The model under review builds one solid part; all positions refer to its coordinate system, in mm. A direction names the side the tool comes from. Coordinates: 2 decimals unless noted, no trailing zeros. Loops run counter-clockwise (first coordinate to the right, second up) from the corner with the lowest first, then second, coordinate; pieces in that order, holes last. Notation, with made-up numbers: M 85.5,-4.75 L 127.5,-4.75 A18 cw 127.5,9.25 Z; hole C 80,12 d6. An arc over 180 degrees is marked long. One line per item, written item: value.
```python
from build123d import *

# Parameters (mm, degrees)
SKETCH_1_W          = 32
SKETCH_1_H          = 35
EXTRUDE_1_DEPTH     = 14
CUT_EXTRUDE_1_REACH = 37
SKETCH_2_R          = 6.1
EXTRUDE_2_DEPTH     = 33
FILLET_1_R          = 3
SKETCH_6_W          = 14
SKETCH_6_H          = 35
EXTRUDE_4_DEPTH     = 4
CUT_EXTRUDE_2_DEPTH = 10
SKETCH_5_W          = 32
SKETCH_5_H          = 4
EXTRUDE_5_DEPTH     = 2
CUT_EXTRUDE_3_REACH = 20
SKETCH_8_R          = 2
CUT_EXTRUDE_4_DEPTH = 3.5


with BuildPart() as part:
    # Эскиз1 → Бобышка-Вытянуть1 (new body)
    with BuildSketch(Plane.XY):
        Rectangle(SKETCH_1_W, SKETCH_1_H)
    extrude(amount=EXTRUDE_1_DEPTH)

    # Эскиз2 → Вырез-Вытянуть1 (cut, up to next)
    with BuildSketch(Plane(origin=(0, 17.5, 0), x_dir=(1, 0, 0), z_dir=(0, 1, 0)), mode=Mode.PRIVATE) as cut_extrude_1_sk1:
        with Locations((-9, -7)):
            Circle(SKETCH_2_R)
    cut_extrude_1_tool1 = extrude(cut_extrude_1_sk1.sketch, amount=-CUT_EXTRUDE_1_REACH, mode=Mode.PRIVATE) & part.part
    add(cut_extrude_1_tool1.solids().sort_by_distance((-9, 17.5, 7))[0], mode=Mode.SUBTRACT)
    # Эскиз2 → Вырез-Вытянуть1 (cut, up to next)
    with BuildSketch(Plane(origin=(0, 17.5, 0), x_dir=(1, 0, 0), z_dir=(0, 1, 0)), mode=Mode.PRIVATE) as cut_extrude_1_sk2:
        with Locations((9, -7)):
            Circle(SKETCH_2_R)
    cut_extrude_1_tool2 = extrude(cut_extrude_1_sk2.sketch, amount=-CUT_EXTRUDE_1_REACH, mode=Mode.PRIVATE) & part.part
    add(cut_extrude_1_tool2.solids().sort_by_distance((9, 17.5, 7))[0], mode=Mode.SUBTRACT)

    # Эскиз3 → Бобышка-Вытянуть2 (add)
    with BuildSketch(Plane(origin=(0, -17.5, 0), x_dir=(1, 0, 0), z_dir=(0, 1, 0))):
        Polygon((-14, -18), (-10, -14), (10, -14), (14, -18), align=None)
    extrude(amount=EXTRUDE_2_DEPTH)

    # Скругление1
    fillet_1_edges = [part.edges().sort_by_distance(p)[0] for p in [
        (-16, 0, 0),
    ]]
    fillet(fillet_1_edges, radius=FILLET_1_R)

    # Эскиз6 → Бобышка-Вытянуть4 (add)
    with BuildSketch(Plane(origin=(16, 0, 0), x_dir=(0, 0, -1), z_dir=(1, 0, 0))):
        with Locations((-7, 0)):
            Rectangle(SKETCH_6_W, SKETCH_6_H)
    extrude(amount=EXTRUDE_4_DEPTH)

    # Эскиз7 → Вырез-Вытянуть2 (cut)
    with BuildSketch(Plane.XY.offset(14)):
        with BuildLine():
            Line((16, -17.5), (17.5, -17.5))
            ThreePointArc((17.5, -17.5), (18, -17), (17.5, -16.5))
            ThreePointArc((17.5, -16.5), (17, -16), (17.5, -15.5))
            ThreePointArc((17.5, -15.5), (18, -15), (17.5, -14.5))
            ThreePointArc((17.5, -14.5), (17, -14), (17.5, -13.5))
            ThreePointArc((17.5, -13.5), (18, -13), (17.5, -12.5))
            ThreePointArc((17.5, -12.5), (17, -12), (17.5, -11.5))
            ThreePointArc((17.5, -11.5), (18, -11), (17.5, -10.5))
            ThreePointArc((17.5, -10.5), (17, -10), (17.5, -9.5))
            ThreePointArc((17.5, -9.5), (18, -9), (17.5, -8.5))
            ThreePointArc((17.5, -8.5), (17, -8), (17.5, -7.5))
            ThreePointArc((17.5, -7.5), (18, -7), (17.5, -6.5))
            ThreePointArc((17.5, -6.5), (17, -6), (17.5, -5.5))
            ThreePointArc((17.5, -5.5), (18, -5), (17.5, -4.5))
            ThreePointArc((17.5, -4.5), (17, -4), (17.5, -3.5))
            ThreePointArc((17.5, -3.5), (18, -3), (17.5, -2.5))
            ThreePointArc((17.5, -2.5), (17, -2), (17.5, -1.5))
            ThreePointArc((17.5, -1.5), (18, -1), (17.5, -0.5))
            ThreePointArc((17.5, -0.5), (17, 0), (17.5, 0.5))
            ThreePointArc((17.5, 0.5), (18, 1), (17.5, 1.5))
            ThreePointArc((17.5, 1.5), (17, 2), (17.5, 2.5))
            ThreePointArc((17.5, 2.5), (18, 3), (17.5, 3.5))
            ThreePointArc((17.5, 3.5), (17, 4), (17.5, 4.5))
            ThreePointArc((17.5, 4.5), (18, 5), (17.5, 5.5))
            ThreePointArc((17.5, 5.5), (17, 6), (17.5, 6.5))
            ThreePointArc((17.5, 6.5), (18, 7), (17.5, 7.5))
            ThreePointArc((17.5, 7.5), (17, 8), (17.5, 8.5))
            ThreePointArc((17.5, 8.5), (18, 9), (17.5, 9.5))
            ThreePointArc((17.5, 9.5), (17, 10), (17.5, 10.5))
            ThreePointArc((17.5, 10.5), (18, 11), (17.5, 11.5))
            ThreePointArc((17.5, 11.5), (17, 12), (17.5, 12.5))
            ThreePointArc((17.5, 12.5), (18, 13), (17.5, 13.5))
            ThreePointArc((17.5, 13.5), (17, 14), (17.5, 14.5))
            ThreePointArc((17.5, 14.5), (18, 15), (17.5, 15.5))
            ThreePointArc((17.5, 15.5), (17, 16), (17.5, 16.5))
            ThreePointArc((17.5, 16.5), (18, 17), (17.5, 17.5))
            Line((17.5, 17.5), (16, 17.5))
            Line((16, 17.5), (16, -17.5))
        make_face()
    extrude(amount=-CUT_EXTRUDE_2_DEPTH, mode=Mode.SUBTRACT)

    # Эскиз5 → Бобышка-Вытянуть5 (add)
    with BuildSketch(Plane(origin=(0, 15.5, 0), x_dir=(-1, 0, 0), z_dir=(0, 1, 0))):
        with Locations((0, 16)):
            Rectangle(SKETCH_5_W, SKETCH_5_H)
    extrude(amount=EXTRUDE_5_DEPTH)

    # Эскиз8 → Вырез-Вытянуть3 (cut, up to next)
    with BuildSketch(Plane.XY.offset(18), mode=Mode.PRIVATE) as cut_extrude_3_sk1:
        Circle(SKETCH_8_R)
    cut_extrude_3_tool1 = extrude(cut_extrude_3_sk1.sketch, amount=-CUT_EXTRUDE_3_REACH, mode=Mode.PRIVATE) & part.part
    add(cut_extrude_3_tool1.solids().sort_by_distance((0, 0, 18))[0], mode=Mode.SUBTRACT)

    # Эскиз9 → Вырез-Вытянуть4 (cut)
    with BuildSketch(Plane(origin=(0, 0, 0), x_dir=(-1, 0, 0), z_dir=(0, 0, -1))):
        Polygon((0, -4.041451884), (3.5, -2.020725942), (3.5, 2.020725942), (0, 4.041451884), (-3.5, 2.020725942), (-3.5, -2.020725942), align=None)
    extrude(amount=-CUT_EXTRUDE_4_DEPTH, mode=Mode.SUBTRACT)


solid = part.part
```
(1) Tool access review of faces 1 (the face through (12, -1, 16)), 2 (the face through (16.8, -3.6, 4)), 3 (the face through (18, 0, 14)), 4 (the face through (-13, -1, 14)), 5 (the face through (3.5, 0, 2)): name each direction out of +Z, -Z, +X, -X, +Y, -Y from which nothing blocks a thin tool from reaching the whole face with its end or side.
Checks:
face 1: +X, -Y
face 2: +Z
face 3: +Z, +X, +Y, -Y
face 4: -X, -Y
face 5: -Z
(2) Add section C-C on z = 2. State the section outline as (x, y) points, then the cut area to 3 significant figures.
Checks:
outline: M -15.83,-17.5 L -12.49,-17.5 L -12.49,17.5 L -15.83,17.5 Z; M -5.51,-17.5 L 5.51,-17.5 L 5.51,17.5 L -5.51,17.5 Z; M 12.49,-17.5 L 20,-17.5 L 20,17.5 L 12.49,17.5 Z; hole M -3.5,-2.02 L 0,-4.04 L 3.5,-2.02 L 3.5,2.02 L 0,4.04 L -3.5,2.02 Z
area: 722 mm^2
(3) Add section A-A on y = -1. State the section outline as (x, z) points.
Checks:
outline: M -16,3 A3 ccw -13,0 L -3.5,0 L -3.5,3.5 L -1.73,3.5 L -1.73,18 L -14,18 L -10,14 L -16,14 Z; M 1.73,3.5 L 3.5,3.5 L 3.5,0 L 20,0 L 20,14 L 18,14 L 18,4 L 16,4 L 16,14 L 10,14 L 14,18 L 1.73,18 Z; hole C -9,7 d12.2; hole C 9,7 d12.2
(4) Add section B-B on x = 0.5. State the section outline as (y, z) points, then the cut area to 3 significant figures.
Checks:
outline: M -17.5,0 L -3.75,0 L -3.75,3.5 L -1.94,3.5 L -1.94,18 L -17.5,18 Z; M 1.94,3.5 L 3.75,3.5 L 3.75,0 L 17.5,0 L 17.5,18 L 1.94,18 Z
area: 548 mm^2
(5) Draft analysis for pull direction Z (two halves, no side actions). For faces 6 (the face through (7, 0, 0)), 7 (the face through (-14, 15.5, 16)), 8 (the face through (14.82, 0.25, 5.17)), 9 (the face through (2, 17.5, 11)), state which applies: pulls with the +Z half, pulls with the -Z half, needs draft (parallel to the pull), parting line crosses it, or undercut.
Checks:
face 6: pulls with the -Z half
face 7: undercut
face 8: undercut
face 9: needs draft
(6) To check wall thickness, follow L1, parallel to X at y = 5, z = 7; L2, parallel to X at y = -4, z = 7; L3, parallel to Y at x = 0, z = 8.75. State the ranges of each line that lie inside material, in increasing order. Write a range as [from, to].
Checks:
L1: [-16, -15.1], [-2.9, 2.9], [15.1, 16], [18, 20]
L2: [-16, -15.1], [-2.9, 2.9], [15.1, 16], [17, 20]
L3: [-17.5, -2], [2, 17.5]
(7) Add section D-D on y = 8. State the section outline as (x, z) points.
Checks:
outline: M -16,3 A3 ccw -13,0 L 20,0 L 20,14 L 17,14 L 17,4 L 16,4 L 16,14 L 10,14 L 14,18 L -14,18 L -10,14 L -16,14 Z; hole C -9,7 d12.2; hole C 9,7 d12.2
(8) Insertion check: pin 1 Ø0.6 at (x, y) = (17.5, -2) entering from +Z; pin 2 Ø3.5 at (x, y) = (-0.5, -1) entering from -Z; pin 3 Ø2 at (x, z) = (14, 15.5) entering from -Y. Each pin has a flat end and moves straight along its axis. Give the tip position at first contact, or say it passes through.
Checks:
pin 1: z = 14
pin 2: z = 3.5
pin 3: y = 15.5
